from build123d import *

# Parameters (mm, degrees)
SKETCH_1_R          = 7.65
EXTRUDE_1_DEPTH     = 10.3
SKETCH_2_R          = 1.5
CUT_EXTRUDE_1_DEPTH = 10.5
CHAMFER_1_SIZE      = 6
FILLET_1_R          = 2
EXTRUDE_START       = 3
SKETCH_4_W          = 7
SKETCH_4_H          = 13.5
EXTRUDE_2_DEPTH     = 9


with BuildPart() as part:
    # ｽｹｯﾁ1 → ﾎﾞｽ - 押し出し1 (new body)
    with BuildSketch(Plane(origin=(0, 0, 0), x_dir=(1, 0, 0), z_dir=(0, 1, 0))):
        with BuildLine():
            Line((17.17, 14.29), (-5.977959518, 14.29))
            ThreePointArc((-5.977959518, 14.29), (-12.244374402, 9.48764436), (-15.33, 2.220630541))
            Line((-15.33, 2.220630541), (-15.33, -2.220630541))
            ThreePointArc((-15.33, -2.220630541), (-12.244374402, -9.48764436), (-5.977959518, -14.29))
            Line((-5.977959518, -14.29), (17.17, -14.29))
            Line((17.17, -14.29), (17.17, 14.29))
        make_face()
        with Locations(Location((0, 0, 0), (0, 0, 90))):
            Circle(SKETCH_1_R, mode=Mode.SUBTRACT)
    extrude(amount=EXTRUDE_1_DEPTH)

    # ｽｹｯﾁ2 → ｶｯﾄ - 押し出し1 (cut)
    with BuildSketch(Plane.XZ):
        with Locations(Location((0, 9.5, 0), (0, 0, 270))):
            Circle(SKETCH_2_R)
        with Locations(Location((0, -9.5, 0), (0, 0, 270))):
            Circle(SKETCH_2_R)
    extrude(amount=-CUT_EXTRUDE_1_DEPTH, mode=Mode.SUBTRACT)

    # 面取り1
    chamfer_1_edges = [part.edges().sort_by_distance(p)[0] for p in [
        (17.17, 5.15, -14.29),
        (17.17, 5.15, 14.29),
    ]]
    chamfer(chamfer_1_edges, length=CHAMFER_1_SIZE)

    # ﾌｨﾚｯﾄ1
    fillet_1_edges = [part.edges().sort_by_distance(p)[0] for p in [
        (11.17, 5.15, -14.29),
        (17.17, 5.15, 8.29),
        (17.17, 5.15, -8.29),
        (11.17, 5.15, 14.29),
    ]]
    fillet(fillet_1_edges, radius=FILLET_1_R)

    # ｽｹｯﾁ4 → ﾎﾞｽ - 押し出し2 (add)
    with BuildSketch(Plane(origin=(0, 0, 0), x_dir=(1, 0, 0), z_dir=(0, 1, 0)).offset(EXTRUDE_START)):
        with Locations((20.67, 0)):
            Rectangle(SKETCH_4_W, SKETCH_4_H)
    extrude(amount=EXTRUDE_2_DEPTH)


solid = part.part
For this review, take the finished solid that the model builds, in its own axes (mm). A direction names the side the tool comes from. Coordinates: 2 decimals unless noted, no trailing zeros. Loops run counter-clockwise (first coordinate to the right, second up) from the corner with the lowest first, then second, coordinate; pieces in that order, holes last. Notation, with made-up numbers: (55, -16) - (95, -16) arc R15 cw to (95, 5) - close; hole circle Ø2 at (38.5, -4.75). An arc over 180 degrees is marked (long way). Use a Markdown table: item, result. Add a question column.
Item 1: We need section D-D (x = -5.5). Give the boundary of the cut face in (y, z), and give its area (3 significant figures).
Item 2: Mouldability with a two-part tool opening along X and no side actions: class faces 1 (the face through (4.655, 5.078, 6.071)), 2 (the face through (-12.31, 5.08, 9.4)), 3 (the face through (0, 5, 11)), 4 (the face through (11.1, 5.22, -14.14)) as pulls with the +X half, pulls with the -X half, needs draft (parallel to the pull), parting line crosses it, or undercut.
Item 3: Tool access review of faces 5 (the face through (21, 7, -6.75)), 6 (the face through (21, 7, 6.75)), 7 (the face through (17.17, 11, 0)), 8 (the face through (2, 5, 14.29)), 9 (the face through (21, 3, 0)): name each direction out of +Z, -Z, +X, -X, +Y, -Y from which nothing blocks a thin tool from reaching the whole face with its end or side.
Item 4: We need section C-C (y = 7.75). Give the boundary of the cut face in (x, z).
Item 5: For line 1 (Z direction, x = 1, y = 10.25); line 2 (Y direction, x = -9, z = 6.5); line 3 (X direction, y = 7.5, z = -3), list the stretches that pass through material, from the lowest coordinate up.
Item 6: We need section B-B (x = 0). Give the boundary of the cut face in (y, z).
Item 7: Insertion check: pin 1 Ø2 at (x, y) = (20, 7) entering from +Z; pin 2 Ø1 at (y, z) = (3, 10) entering from +X; pin 3 Ø1 at (y, z) = (2.5, 11.5) entering from +X; pin 4 Ø2.5 at (x, z) = (0, -9.5) entering from +Y (3 decimals). Each pin has a flat end and moves straight along its axis. Give the tip position at first contact, or say it passes through.
Item 8: We need section A-A (z = 0). Give the boundary of the cut face in (x, y).
Results list:
| question | item | result |
|---|---|---|
| 1 | outline | (0, -14.29) - (10.3, -14.29) - (10.3, -5.32) - (0, -5.32) - close; (0, 5.32) - (10.3, 5.32) - (10.3, 14.29) - (0, 14.29) - close |
| 1 | area | 185 mm^2 |
| 2 | face 1 | undercut |
| 2 | face 2 | pulls with the -X half |
| 2 | face 3 | undercut |
| 2 | face 4 | pulls with the +X half |
| 3 | face 5 | -Z, +X, +Y, -Y |
| 3 | face 6 | +Z, +X, +Y, -Y |
| 3 | face 7 | +Z, -Z, -X, +Y |
| 3 | face 8 | +Z, +X, -X, +Y, -Y |
| 3 | face 9 | +Z, -Z, +X, -Y |
| 4 | outline | (-15.33, -2.22) arc R15.49 ccw to (-5.98, -14.29) - (10.34, -14.29) arc R2 ccw to (11.76, -13.7) - (16.58, -8.88) arc R2 ccw to (17.17, -7.46) - (17.17, -6.75) - (24.17, -6.75) - (24.17, 6.75) - (17.17, 6.75) - (17.17, 7.46) arc R2 ccw to (16.58, 8.88) - (11.76, 13.7) arc R2 ccw to (10.34, 14.29) - (-5.98, 14.29) arc R15.49 ccw to (-15.33, 2.22) - close; hole circle Ø15.3 at (0, 0); hole circle Ø3 at (0, -9.5); hole circle Ø3 at (0, 9.5) |
| 5 | line 1 | z = -14.29 to -10.62, -8.38 to -7.58, 7.58 to 8.38, 10.62 to 14.29 |
| 5 | line 2 | y = 0 to 10.3 |
| 5 | line 3 | x = -15.2 to -7.04, 7.04 to 24.17 |
| 6 | outline | (0, -14.29) - (10.3, -14.29) - (10.3, -11) - (0, -11) - close; (0, -8) - (10.3, -8) - (10.3, -7.65) - (0, -7.65) - close; (0, 7.65) - (10.3, 7.65) - (10.3, 8) - (0, 8) - close; (0, 11) - (10.3, 11) - (10.3, 14.29) - (0, 14.29) - close |
| 7 | pin 1 | stops at z = 6.75 |
| 7 | pin 2 | stops at x = 15.96 |
| 7 | pin 3 | stops at x = 14.46 |
| 7 | pin 4 | passes through |
| 8 | outline | (-15.33, 0) - (-7.65, 0) - (-7.65, 10.3) - (-15.33, 10.3) - close; (7.65, 0) - (17.17, 0) - (17.17, 3) - (24.17, 3) - (24.17, 12) - (17.17, 12) - (17.17, 10.3) - (7.65, 10.3) - close |
